```python
from build123d import *

# Parameters (mm, degrees)
F0_R     = 11.05
F1_DEPTH = 7


# Not quite as in the source:
# - a feature names something its author has since deleted; it is built from what else it names


with BuildPart() as f1:
    # F0 (on Top) → F1 (new body)
    with BuildSketch(Plane.XY):
        with BuildLine():
            ThreePointArc((-4.0106673609, 13.4132228536), (4.561996815, 13.2358673709), (11.4233995183, 8.0935742071))
            ThreePointArc((11.4233995183, 8.0935742071), (10.0789971933, 13.6745719731), (12.9496720608, 18.6459077574))
            ThreePointArc((12.9496720608, 18.6459077574), (15.9741224369, 25.5738093143), (11.8787878788, 31.9276549937))
            ThreePointArc((11.8787878788, 31.9276549937), (-8.2529606774, 33.568130398), (-22.7753295029, 19.5296382006))
            ThreePointArc((-22.7753295029, 19.5296382006), (-21.7981073273, 16.9621679379), (-19.1543041216, 17.7086070442))
            ThreePointArc((-19.1543041216, 17.7086070442), (-12.9655505969, 23.1890748663), (-4.7818295921, 24.3565114828))
            ThreePointArc((-4.7818295921, 24.3565114828), (-0.0139046539, 19.1936864048), (-4.0106673609, 13.4132228536))
        make_face()
        with BuildLine():
            ThreePointArc((13.6215254183, -3.2332716061), (13.9050594363, -1.6276738223), (14, 0))
            ThreePointArc((14, 0), (13.3403072164, 4.2469051522), (11.4233995183, 8.0935742071))
            ThreePointArc((11.4233995183, 8.0935742071), (4.561996815, 13.2358673709), (-4.0106673609, 13.4132228536))
            ThreePointArc((-4.0106673609, 13.4132228536), (-9.1815989768, 10.5687388192), (-12.7209406299, 5.8461670769))
            ThreePointArc((-12.7209406299, 5.8461670769), (-13.7435957918, -2.6671285517), (-9.6108580574, -10.1799512475))
            ThreePointArc((-9.6108580574, -10.1799512475), (-4.561996815, -13.2358673709), (1.2975411116, -13.939741284))
            ThreePointArc((1.2975411116, -13.939741284), (9.1815989768, -10.5687388192), (13.6215254183, -3.2332716061))
        make_face()
        Circle(F0_R, mode=Mode.SUBTRACT)
        with BuildLine():
            ThreePointArc((-9.6108580574, -10.1799512475), (-13.7435957918, -2.6671285517), (-12.7209406299, 5.8461670769))
            ThreePointArc((-12.7209406299, 5.8461670769), (-16.8820253112, 1.8913816276), (-22.6226658249, 1.8917910967))
            ThreePointArc((-22.6226658249, 1.8917910967), (-30.1346297562, 1.0470911764), (-33.5895542472, -5.6764954277))
            ThreePointArc((-33.5895542472, -5.6764954277), (-24.9443733435, -23.931338802), (-5.5254980569, -29.4888330294))
            ThreePointArc((-5.5254980569, -29.4888330294), (-3.7906146738, -27.3587986688), (-5.7589515051, -25.4424174832))
            ThreePointArc((-5.7589515051, -25.4424174832), (-13.5995526261, -22.8230336242), (-18.7024428957, -16.3194416447))
            ThreePointArc((-18.7024428957, -16.3194416447), (-16.6152676918, -9.6088849859), (-9.6108580574, -10.1799512475))
        make_face()
        with BuildLine():
            ThreePointArc((23.4842724877, -8.0370698381), (16.6291723457, -9.5848014189), (13.6215254183, -3.2332716061))
            ThreePointArc((13.6215254183, -3.2332716061), (9.1815989768, -10.5687388192), (1.2975411116, -13.939741284))
            ThreePointArc((1.2975411116, -13.939741284), (6.8030281179, -15.5659536006), (9.6729937641, -20.537698854))
            ThreePointArc((9.6729937641, -20.537698854), (14.1605073193, -26.6209004907), (21.7107663685, -26.2511595661))
            ThreePointArc((21.7107663685, -26.2511595661), (33.1973340209, -9.6367915959), (28.3008275599, 9.9591948288))
            ThreePointArc((28.3008275599, 9.9591948288), (25.5887220011, 10.3966307309), (24.9132556267, 7.733810439))
            ThreePointArc((24.9132556267, 7.733810439), (26.565103223, -0.3660412422), (23.4842724877, -8.0370698381))
        make_face()
    extrude(amount=F1_DEPTH)


solid = f1.part
```
CAD build for the part. Positions are in the model's coordinates, mm. A direction names the side the tool comes from. Give positions to 0.01 mm unless a question says otherwise; leave off trailing zeros. Order: outer loops, then holes, each group sorted by start corner. A loop starts at its lowest first (then second) coordinate and runs counter-clockwise, first axis right, second up.
(1) Saw through at A-A, the plane x = 3.5. Give the cut face in (y, z).
(2) Saw through at D-D, the plane y = 30. Give the cut face in (x, z), then the cut area to 3 significant figures.
(3) Saw through at C-C, the plane z = 6.25. Give the cut face in (x, y), then the cut area to 3 significant figures.
(4) Drill centre lines: L1, parallel to X at y = -9.5, z = 1.25; L2, parallel to X at y = 4, z = 5.5; L3, parallel to X at y = -5, z = 3.5. Where is each one in solid material? Low to high.
(5) Tool access for faces 4 (the cylindrical face through (-13.07, 23.14, 3.45)), 5 (the flat face through (-0.5, -11.3, 0)), 6 (the cylindrical face through (-9.12, 10.62, 3.45)): list every direction of +Z, -Z, +X, -X, +Y, -Y with a clear straight run to the whole face (end or side of a thin tool).
(6) Saw through at B-B, the plane y = -24.5. Give the cut face in (x, z), then the cut area to 3 significant figures.
(7) Mould opens along X. For faces 1 (the cylindrical face through (6.738, -15.515, 3.451)), 2 (the flat face through (-0.5, -11.3, 7)), 3 (the cylindrical face through (-7.978, 33.665, 3.451)) say: released by +X, released by -X, zero draft, split by the parting line, or undercut.
(8) Flat gauge pins, fed straight in: pin 1 (20 mm diameter, centred on x = 0, y = 0, fed in from +Z); pin 2 (1.5 mm diameter, centred on x = -12.5, z = 5, fed in from -Y). Where does each tip first touch, or does it go through?
Results found:
1. outline: (-14.05, 0) - (-10.48, 0) - (-10.48, 7) - (-14.05, 7) - close; (10.48, 0) - (34.75, 0) - (34.75, 7) - (10.48, 7) - close
2. outline: (-14.83, 0) - (14.19, 0) - (14.19, 7) - (-14.83, 7) - close
2. area: 203 mm2
3. outline: (-33.59, -5.68) arc R24.5 ccw to (-5.53, -29.49) arc R2.03 ccw to (-5.76, -25.44) arc R14.38 cw to (-18.7, -16.32) arc R5.62 cw to (-9.61, -10.18) arc R14 ccw to (1.3, -13.94) arc R7.74 cw to (9.67, -20.54) arc R8 ccw to (21.71, -26.25) arc R24.5 ccw to (28.3, 9.96) arc R2.03 ccw to (24.91, 7.73) arc R14.38 cw to (23.48, -8.04) arc R5.62 cw to (13.62, -3.23) arc R14 ccw to (11.42, 8.09) arc R7.74 cw to (12.95, 18.65) arc R8 ccw to (11.88, 31.93) arc R24.5 ccw to (-22.78, 19.53) arc R2.03 ccw to (-19.15, 17.71) arc R14.38 cw to (-4.78, 24.36) arc R5.62 cw to (-4.01, 13.41) arc R14 ccw to (-12.72, 5.85) arc R7.74 cw to (-22.62, 1.89) arc R8 ccw to start; hole circle Ø22.1 at (0, 0)
3. area: 1,710 mm2
4. L1: x = -33.22 to -16.45, -10.49 to -5.64, 5.64 to 16.46, 21.72 to 33.22
4. L2: x = -13.91 to -10.3, 10.3 to 13.42, 26.29 to 31.78
4. L3: x = -33.57 to -9.85, 9.85 to 13.49, 25.34 to 33.59
5. face 4: +Z, -Z
5. face 5: -Z, +X, -X, +Y, -Y
5. face 6: +Z, -Z, -X
6. outline: (-24.25, 0) - (-10.45, 0) - (-10.45, 7) - (-24.25, 7) - close; (11.43, 0) - (24.25, 0) - (24.25, 7) - (11.43, 7) - close
6. area: 186 mm2
7. face 1: undercut
7. face 2: zero draft
7. face 3: split by the parting line
8. pin 1: passes through
8. pin 2: stops at y = -29.61
